For this review, take the finished solid that the model builds, in its own axes (mm). Give positions to 0.01 mm unless a question says otherwise; leave off trailing zeros. Answer as a JSON object with one key per item and string values. Group by question number.
from build123d import *

# Parameters (mm, degrees)
F1_DEPTH = 3.175
F2_R     = 5


# Not quite as in the source:
# - a length typed as a fraction of an inch, garbled in the dataset ("3 / 203.2 mm" for 3/8 in), is restored


with BuildPart() as f1:
    # F0 (on Front) → F1 (new body)
    with BuildSketch(Plane.XZ):
        with BuildLine():
            ThreePointArc((6, 0), (5.7619448426, 1.6733175524), (5.0666694563, 3.2138544803))
            ThreePointArc((5.0666694563, 3.2138544803), (0.0307741544, 5.9999210788), (-5.0334354285, 3.2656588595))
            ThreePointArc((-5.0334354285, 3.2656588595), (-5.2722838105, -2.8640920763), (0, -6))
            add(Edge.make_bspline(
                [(0, -6), (0.7881316779, -5.8923160671), (1.5037462454, -5.7565864603), (2.1584342276, -5.5983177549)],
                knots=[0, 0, 0, 0, 0.0486422356, 0.0486422356, 0.0486422356, 0.0486422356], degree=3))
            ThreePointArc((2.1584342276, -5.5983177549), (3.7803533787, -4.6592841008), (5.0334354285, -3.2656588595))
            ThreePointArc((5.0334354285, -3.2656588595), (5.7532865638, -1.7028487057), (6, 0))
        make_face()
        with BuildLine():
            ThreePointArc((1.9898590203, 1.3079803675), (2.281304819, 0.6826418425), (2.38125, 0))
            ThreePointArc((2.38125, 0), (-2.281304819, -0.6826418425), (1.9898590203, 1.3079803675))
        make_face(mode=Mode.SUBTRACT)
        with BuildLine():
            add(Edge.make_bspline(
                [(5.0666694563, 3.2138544803), (8.837595406, 5.414485816), (14.2440437805, 6.8995614863), (24.1781340673, 4.7387528577), (32.5091555715, 0)],
                knots=[0.1268767178, 0.1268767178, 0.1268767178, 0.1268767178, 0.46554979, 1, 1, 1, 1], degree=3))
            ThreePointArc((5.0666694563, 3.2138544803), (5.7619448426, 1.6733175524), (6, 0))
            ThreePointArc((6, 0), (5.7532865638, -1.7028487057), (5.0334354285, -3.2656588595))
            ThreePointArc((5.0334354285, -3.2656588595), (3.7803533787, -4.6592841008), (2.1584342276, -5.5983177549))
            add(Edge.make_bspline(
                [(2.1584342276, -5.5983177549), (7.8149044031, -4.2308843573), (10.3239452596, 2.6732879939), (27.8337137958, 0), (30.8784303042, -3.806720163)],
                knots=[0.0486422356, 0.0486422356, 0.0486422356, 0.0486422356, 0.4689086255, 1, 1, 1, 1], degree=3))
            Line((30.8784303042, -3.806720163), (32.5091555715, 0))
        make_face()
        with BuildLine():
            add(Edge.make_bspline(
                [(0, -6), (0.7881316779, -5.8923160671), (1.5037462454, -5.7565864603), (2.1584342276, -5.5983177549)],
                knots=[0, 0, 0, 0, 0.0486422356, 0.0486422356, 0.0486422356, 0.0486422356], degree=3))
            ThreePointArc((0, -6), (1.0977462071, -5.8987247151), (2.1584342276, -5.5983177549))
        make_face()
    extrude(amount=F1_DEPTH)

    # F2
    f2_edges = [f1.edges().sort_by_distance(p)[0] for p in [
        (5.066669, -1.5875, 3.213854),
    ]]
    fillet(f2_edges, radius=F2_R)


solid = f1.part
1) For pin 1 (1 mm diameter, centred on y = -1, z = -2.5, fed in from -X); pin 2 (1 mm diameter, centred on x = 27.5, y = -2, fed in from -Z), all flat-tipped, find the tip position at first contact; note any pin that passes through.
2) For line 1 (X direction, y = -1.2, z = 1.75); line 2 (X direction, y = -0.6, z = -1.75); line 3 (X direction, y = -1.75, z = -3.25), list the stretches that pass through material, from the lowest coordinate up.
3) Consider section A-A (z = -0.75). Give the number of separate pieces and of enclosed holes in the cut face, plus the area to 3 significant figures.
Result set:
{
 "1": {"pin 1": "stops at x = -5.66", "pin 2": "stops at z = -1.63"},
 "2": {"line 1": "x = -5.74 to -1.61, 1.61 to 29.23", "line 2": "x = -5.74 to -1.61, 1.61 to 9.51, 28.23 to 31.76", "line 3": "x = -5.04 to 7.43, 30.37 to 31.12"},
 "3": {"separate pieces": "3", "enclosed holes": "0", "area": "59.9 mm2"}
}
